Autodesk Inventor part; units mm, degrees
ref_plane "YZ Plane" through (0, 0, 0) normal (1, 0, 0) x (0, 1, 0)
ref_plane "XZ Plane" through (0, 0, 0) normal (0, 1, 0) x (-1, 0, 0)
ref_plane "XY Plane" through (0, 0, 0) normal (0, 0, 1) x (1, 0, 0)
sketch "Sketch1" plane through (0, 0, 0) normal (0, 1, 0) x (-1, 0, 0)
  circle A0 centre (0, 0) radius 14
  line L0 (0.7278, -24) -> (-0.7278, -24)
  line L1 (-0.7278, 24) -> (0.7278, 24)
  line L2 (16.75, 0) -> (0, 0) construction
  line L3 (0, 24) -> (0, 0) construction
  line L4 (0, 0) -> (0, -24) construction
  line L5 (-28.5847, 0) -> (0, 0) construction
  line L6 (9.7305, 18.3534) -> (15.0795, 7.2919)
  line L7 (9.7305, -18.3534) -> (15.0795, -7.2919)
  line L8 (-9.7305, 18.3534) -> (-15.0795, 7.2919)
  line L9 (-9.7305, -18.3534) -> (-15.0795, -7.2919)
  arc A1 (-15.0795, 7.2919) -> (-15.0795, -7.2919) centre (0, 0) ccw
  arc A2 (15.0795, -7.2919) -> (15.0795, 7.2919) centre (0, 0) ccw
  arc A3 (9.7305, 18.3534) -> (0.7278, 24) centre (0.7278, 14) ccw
  arc A4 (-0.7278, 24) -> (-9.7305, 18.3534) centre (-0.7278, 14) ccw
  arc A5 (0.7278, -24) -> (9.7305, -18.3534) centre (0.7278, -14) ccw
  arc A6 (-9.7305, -18.3534) -> (-0.7278, -24) centre (-0.7278, -14) ccw
  point P0 (-7, 24)
  point P1 (7, 24)
  dimension "d0" = 28
  dimension "d3" = 16.75
  dimension "d4" = 48
  dimension "d5" = 14
  dimension "d6" = 10
extrude "Extrusion1" add sketch "Sketch1" along normal blind 2
sketch "Sketch2" plane through (0, 2, 0) normal (0, 1, 0) x (1, 0, 0)
  circle A0 centre (0, 0) radius 15
  circle A1 centre (0, 0) radius 14
  circle A2 centre (0, 0) radius 14 construction
  dimension "d9" = 30
extrude "Extrusion2" add sketch "Sketch2" along normal blind 117
sketch "Sketch5" plane through (0, 0, 0) normal (1, 0, 0) x (0, 1, 0)
  line L0 (0, 14) -> (119, 14) construction
  line L1 (118.2507, 14) -> (121.1776, 4)
  line L2 (2, 15) -> (119, 15) construction
  line L3 (119, 15) -> (122, 4.75)
  line L4 (0, 0) -> (118.2507, 0) construction
  line L5 (118.2507, 0) -> (118.2507, 14) construction
  line L6 (122, 4.75) -> (129, 4.75)
  line L7 (129, 4.75) -> (129, 3.75)
  line L8 (129, 3.75) -> (124, 3.75)
  line L9 (124, 3.75) -> (124, 1.75)
  line L10 (124, 1.75) -> (131.2, 1.75)
  line L11 (131.2, 1.75) -> (131.2, 1.25)
  line L12 (131.2, 1.25) -> (122.1776, 1.25)
  line L13 (121.1776, 4) -> (122.1776, 4)
  line L14 (122.1776, 4) -> (122.1776, 1.25)
  line L15 (119, 15) -> (119, 14)
  line L16 (119, 14) -> (118.2507, 14)
  dimension "d20" = 1
  dimension "d21" = 4.75
  dimension "d22" = 3
  dimension "d23" = 1
  dimension "d24" = 7
  dimension "d25" = 2.2
  dimension "d26" = 2
  dimension "d27" = 1.25
  dimension "d28" = 5
  dimension "d29" = 4
  dimension "d31" = 1
revolve "Revolution2" add sketch "Sketch5" angle 360 about axis through (0, 0, 0) along (0, 1, 0)
sketch "Sketch6" plane through (0, 0, 0) normal (0, -1, 0) x (1, 0, 0)
  circle A0 centre (0, -20) radius 1.75
  line L0 (0, -20) -> (0, 0) construction
  dimension "d33" = 3.5
  dimension "d34" = 20
extrude "Extrusion4" cut sketch "Sketch6" against normal up to surface (2 mm away)
properties part number "CH_01_0006_syringe"
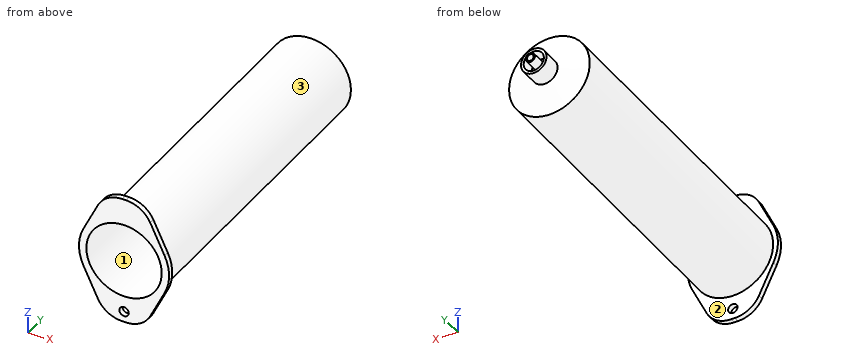
Could you check a few things on this model? Use its own coordinates, in mm. Face numbers are marked on the shaded views. Round coordinates to 2 decimals unless told otherwise and drop trailing zeros. Loops run counter-clockwise (first coordinate to the right, second up) from the corner with the lowest first, then second, coordinate; pieces in that order, holes last. Notation, with made-up numbers: (67.5, 16) - (105.5, 16) arc R17 ccw to (105.5, 21) - close; hole circle Ø1 at (-26.75, -35.75). An arc over 180 degrees is marked (long way). Write item = value, one per line.
1) I'm going to push flat-ended pins straight in: P1, Ø10, axis at x = -6, y = 63, coming from the -Z side; P2, Ø1, axis at y = 114, z = -9, coming from the -X side; P3, Ø3, axis at x = -3.5, y = 96.5, coming from the -Z side; P4, Ø1.5, axis at x = 0, z = 0, coming from the -Y side. Where does each tip first touch, or does it pass through?
Computed:
P1 = -14.97
P2 = -12.36
P3 = -14.87
P4 = through
2) Imagine slicing it at A-A (z = -20). Please give me the cut outline in (x, y), and give its area (3 significant figures).
Computed:
outline = (-8.73, 0) - (-1.75, 0) - (-1.75, 2) - (-8.73, 2) - close; (1.75, 0) - (8.73, 0) - (8.73, 2) - (1.75, 2) - close
area = 27.9 mm2
3) Imagine slicing it at B-B (y = 94.5). Please give me the cut outline in (x, z).
Computed:
outline = circle Ø30 at (0, 0); hole circle Ø28 at (0, 0)
4) If we mould it in two halves opening along Z, with no side actions, what happens to the marked faces 1, 2 and 3? For each: pulls with the +Z half, pulls with the -Z half, needs draft (parallel to the pull), parting line crosses it, or undercut.
Computed:
face_1 = undercut
face_2 = needs draft
face_3 = parting line crosses it
5) I need wall thicknesses on line 1 along X through (y, z) = (126, 0); line 2 along X through (y, z) = (122.05, 0); line 3 along X through (y, z) = (57, 0). Which ranges of each line are inside material? Lowest first, please. Write a range as from..to.
Computed:
line_1 = -4.75..-3.75, -1.75..-1.25, 1.25..1.75, 3.75..4.75
line_2 = -4.75..-4, 4..4.75
line_3 = -15..-14, 14..15
